Geometry: final body of the model. Coordinates: model frame, mm. A direction names the side the tool comes from. Round coordinates to 2 decimals unless told otherwise and drop trailing zeros. Loops run counter-clockwise (first coordinate to the right, second up) from the corner with the lowest first, then second, coordinate; pieces in that order, holes last. Notation, with made-up numbers: M 44.25,66.25 L 75.25,66.25 A18 cw 75.25,93.25 Z; hole C 16.5,-40 d6. An arc over 180 degrees is marked long. Answer as a JSON object with one key per item and string values.
```python
from build123d import *

# Parameters (mm, degrees)
BOSS_EXTRUDE1_DEPTH      = 30
BOSS_EXTRUDE2_DEPTH      = 14
BOSS_EXTRUDE2_DEPTH_BACK = 30
SKETCH2_W                = 14
SKETCH2_H                = 40
SKETCH3_W                = 14
SKETCH3_H                = 20
CUT_EXTRUDE1_DEPTH       = 14
CUT_EXTRUDE2_DEPTH       = 20
CUT_EXTRUDE2_DEPTH_BACK  = 20
SKETCH5_R                = 5
SKETCH6_W                = 10
SKETCH6_H                = 10
BOSS_EXTRUDE3_DEPTH      = 10
CUT_EXTRUDE3_DEPTH       = 15
CUT_EXTRUDE3_DEPTH_BACK  = 5
SKETCH7_R                = 2.5
SKETCH8_W                = 10
SKETCH8_H                = 30
BOSS_EXTRUDE4_DEPTH      = 10
SKETCH9_W                = 5
SKETCH9_H                = 30
CUT_EXTRUDE4_DEPTH       = 10
SKETCH10_R               = 10
CUT_EXTRUDE5_DEPTH       = 5
SKETCH11_R               = 12
CUT_EXTRUDE6_DEPTH       = 5
FILLET1_R                = 7
FILLET3_R                = 5
FILLET2_R                = 2.5


# Some blends are built 0.0001 mm under size
with BuildPart() as part:
    # Sketch1 → Boss-Extrude1 (new body)
    with BuildSketch(Plane(origin=(0, 0, 0), x_dir=(1, 0, 0), z_dir=(0, 1, 0))):
        with BuildLine():
            Line((0, 100), (0, 90))
            ThreePointArc((0, 90), (-90, 0), (0, -90))
            Line((0, -90), (0, -100))
            ThreePointArc((0, -100), (-100, 0), (0, 100))
        make_face()
    extrude(amount=BOSS_EXTRUDE1_DEPTH)

    # Sketch2 → Boss-Extrude2 (add, two sides: drawn at the far end of the back side and taken through both)
    with BuildSketch(Plane.XZ.offset(-BOSS_EXTRUDE2_DEPTH_BACK)):
        with Locations((-97, 0)):
            Rectangle(SKETCH2_W, SKETCH2_H)
    extrude(amount=BOSS_EXTRUDE2_DEPTH + BOSS_EXTRUDE2_DEPTH_BACK)

    # Sketch3 → Cut-Extrude1 (cut)
    with BuildSketch(Plane.XZ.offset(14)):
        with Locations((-97, 0)):
            Rectangle(SKETCH3_W, SKETCH3_H)
    extrude(amount=-CUT_EXTRUDE1_DEPTH, mode=Mode.SUBTRACT)

    # Sketch5 → Cut-Extrude2 (cut, two sides: drawn at the far end of the back side and taken through both)
    with BuildSketch(Plane.XY.offset(-CUT_EXTRUDE2_DEPTH_BACK)):
        with Locations((-97, -7)):
            Circle(SKETCH5_R)
    extrude(amount=CUT_EXTRUDE2_DEPTH + CUT_EXTRUDE2_DEPTH_BACK, mode=Mode.SUBTRACT)

    # Sketch6 → Boss-Extrude3 (add)
    with BuildSketch(Plane(origin=(0, 0, 0), x_dir=(0, 0, -1), z_dir=(1, 0, 0))):
        with Locations((95, 25)):
            Rectangle(SKETCH6_W, SKETCH6_H)
        with Locations((95, 5)):
            Rectangle(SKETCH6_W, SKETCH6_H)
    extrude(amount=BOSS_EXTRUDE3_DEPTH)

    # Sketch7 → Cut-Extrude3 (cut, two sides: drawn at the far end of the back side and taken through both)
    with BuildSketch(Plane(origin=(0, 10, 0), x_dir=(1, 0, 0), z_dir=(0, 1, 0)).offset(-CUT_EXTRUDE3_DEPTH_BACK)):
        with Locations(Location((5, 95, 0), (0, 0, 90))):
            Circle(SKETCH7_R)
    extrude(amount=CUT_EXTRUDE3_DEPTH + CUT_EXTRUDE3_DEPTH_BACK, mode=Mode.SUBTRACT)

    # Sketch8 → Boss-Extrude4 (add)
    with BuildSketch(Plane(origin=(0, 0, 0), x_dir=(0, 0, -1), z_dir=(1, 0, 0))):
        with Locations((-95, 15)):
            Rectangle(SKETCH8_W, SKETCH8_H)
    extrude(amount=BOSS_EXTRUDE4_DEPTH)

    # Sketch9 → Cut-Extrude4 (cut)
    with BuildSketch(Plane(origin=(10, 0, 0), x_dir=(0, 0, -1), z_dir=(1, 0, 0))):
        with Locations((-95, 15)):
            Rectangle(SKETCH9_W, SKETCH9_H)
    extrude(amount=-CUT_EXTRUDE4_DEPTH, mode=Mode.SUBTRACT)

    # Sketch10 → Cut-Extrude5 (cut)
    with BuildSketch(Plane.ZY.offset(104)):
        with Locations((0, 15)):
            Circle(SKETCH10_R)
    extrude(amount=-CUT_EXTRUDE5_DEPTH, mode=Mode.SUBTRACT)

    # Sketch11 → Cut-Extrude6 (cut)
    with BuildSketch(Plane.ZY.offset(99)):
        with Locations((0, 15)):
            Circle(SKETCH11_R)
    extrude(amount=-CUT_EXTRUDE6_DEPTH, mode=Mode.SUBTRACT)

    # Fillet1
    fillet1_edges = [part.edges().sort_by_distance(p)[0] for p in [
        (-104, -14, -15),
        (-90, -14, -15),
        (-104, -14, 15),
        (-90, -14, 15),
    ]]
    fillet(fillet1_edges, radius=FILLET1_R - 0.0001)  # a hair under: the kernel refuses the full size

    # Fillet3
    fillet3_edges = [part.edges().sort_by_distance(p)[0] for p in [
        (10, 5, -90),
        (10, 5, -100),
        (10, 25, -100),
        (10, 25, -90),
    ]]
    fillet(fillet3_edges, radius=FILLET3_R - 0.0001)  # a hair under: the kernel refuses the full size

    # Fillet2
    # the kernel refuses this fillet: 2.5 mm, written as the material it takes off along each edge
    with BuildSketch(Plane(origin=(0, 0, 90), x_dir=(0, 0, 1), z_dir=(1, 0, 0)), Plane(origin=(0, 30, 90), x_dir=(0, -1, 0), z_dir=(1, 0, 0))) as fillet2_piece_1:
        with BuildLine():
            CenterArc((FILLET2_R, -FILLET2_R), FILLET2_R, 90, 90)
            Line((0, -FILLET2_R), (0, 0))
            Line((0, 0), (FILLET2_R, 0))
        make_face()
    extrude(amount=16.25, mode=Mode.SUBTRACT)
    with BuildSketch(Plane(origin=(0, 0, -90), x_dir=(0, 0, -1), z_dir=(1, 0, 0)), Plane(origin=(0, 30, -90), x_dir=(0, -1, 0), z_dir=(1, 0, 0)), Plane(origin=(0, 30, -100), x_dir=(0, 0, 1), z_dir=(1, 0, 0))) as fillet2_piece_2:
        with BuildLine():
            CenterArc((FILLET2_R, FILLET2_R), FILLET2_R, 180, 90)
            Line((0, FILLET2_R), (0, 0))
            Line((0, 0), (FILLET2_R, 0))
        make_face()
    extrude(amount=5.0001, mode=Mode.SUBTRACT)
    with BuildSketch(Plane(origin=(0, 0, 0), x_dir=(0, 0, 1), z_dir=(1, 0, 0))) as fillet2_piece_3_section:
        with BuildLine():
            CenterArc((90 + FILLET2_R, -FILLET2_R), FILLET2_R, 90, 90)
            Line((90, -FILLET2_R), (90, 0))
            Line((90, 0), (90 + FILLET2_R, 0))
        make_face()
    fillet2_piece_3 = revolve(axis=Axis((0, 0, 0), (0, -1, 0)), revolution_arc=180, mode=Mode.PRIVATE)
    fillet2_piece_3 = split(fillet2_piece_3, bisect_by=Plane(origin=(-90, 0.417646948, 90.51789801), z_dir=(1, 0, 0)), keep=Keep.TOP, mode=Mode.PRIVATE)
    add(fillet2_piece_3, mode=Mode.SUBTRACT)
    with BuildSketch(Plane(origin=(0, 0, 0), x_dir=(0, 0, 1), z_dir=(1, 0, 0))) as fillet2_piece_4_section:
        with BuildLine():
            CenterArc((90 + FILLET2_R, -FILLET2_R), FILLET2_R, 90, 90)
            Line((90, -FILLET2_R), (90, 0))
            Line((90, 0), (90 + FILLET2_R, 0))
        make_face()
    fillet2_piece_4 = revolve(axis=Axis((0, 0, 0), (0, -1, 0)), revolution_arc=180, mode=Mode.PRIVATE)
    fillet2_piece_4 = split(fillet2_piece_4, bisect_by=Plane(origin=(-90.062527527, 0.003732432, 20), z_dir=(0, 0, 1)), keep=Keep.TOP, mode=Mode.PRIVATE)
    add(fillet2_piece_4, mode=Mode.SUBTRACT)
    with BuildSketch(Plane(origin=(0, 0, 0), x_dir=(0, 0, 1), z_dir=(1, 0, 0))) as fillet2_piece_5_section:
        with BuildLine():
            CenterArc((90 + FILLET2_R, -FILLET2_R), FILLET2_R, 90, 90)
            Line((90, -FILLET2_R), (90, 0))
            Line((90, 0), (90 + FILLET2_R, 0))
        make_face()
    fillet2_piece_5 = revolve(axis=Axis((0, 0, 0), (0, -1, 0)), revolution_arc=180, mode=Mode.PRIVATE)
    fillet2_piece_5 = split(fillet2_piece_5, bisect_by=Plane(origin=(-90.540406948, 0.460795961, -10), z_dir=(0, 0, 1)), keep=Keep.TOP, mode=Mode.PRIVATE)
    fillet2_piece_5 = split(fillet2_piece_5, bisect_by=Plane(origin=(-90.540406948, 0.460795961, 10), z_dir=(0, 0, -1)), keep=Keep.TOP, mode=Mode.PRIVATE)
    add(fillet2_piece_5, mode=Mode.SUBTRACT)
    with BuildSketch(Plane(origin=(0, 0, 0), x_dir=(0, 0, 1), z_dir=(1, 0, 0))) as fillet2_piece_6_section:
        with BuildLine():
            CenterArc((90 + FILLET2_R, -FILLET2_R), FILLET2_R, 90, 90)
            Line((90, -FILLET2_R), (90, 0))
            Line((90, 0), (90 + FILLET2_R, 0))
        make_face()
    fillet2_piece_6 = revolve(axis=Axis((0, 0, 0), (0, -1, 0)), revolution_arc=180, mode=Mode.PRIVATE)
    fillet2_piece_6 = split(fillet2_piece_6, bisect_by=Plane(origin=(-90.062527448, 0.003732432, -20), z_dir=(0, 0, -1)), keep=Keep.TOP, mode=Mode.PRIVATE)
    add(fillet2_piece_6, mode=Mode.SUBTRACT)
    with BuildSketch(Plane(origin=(0, 30, 0), x_dir=(0, 0, -1), z_dir=(1, 0, 0))) as fillet2_piece_7:
        with BuildLine():
            CenterArc((90 + FILLET2_R, -FILLET2_R), FILLET2_R, 90, 90)
            Line((90 + FILLET2_R, 0), (90, 0))
            Line((90, 0), (90, -FILLET2_R))
        make_face()
    revolve(axis=Axis((0, 30, 0), (0, 1, 0)), revolution_arc=180, mode=Mode.SUBTRACT)
    with BuildSketch(Plane(origin=(0, 0, 0), x_dir=(-0.9903773605712586, 0, -0.1383932211775821), z_dir=(-0.1383932211775821, 0, 0.9903773605712586))) as fillet2_piece_8_section:
        with BuildLine():
            CenterArc((100 - FILLET2_R, -FILLET2_R), FILLET2_R, 0, 90)
            Line((100, -FILLET2_R), (100, 0))
            Line((100, 0), (100 - FILLET2_R, 0))
        make_face()
    fillet2_piece_8 = revolve(axis=Axis((0, 0, 0), (0, -1, 0)), revolution_arc=82.045120461, mode=Mode.PRIVATE)
    fillet2_piece_8 = split(fillet2_piece_8, bisect_by=Plane(origin=(-62.807815321, 0.692124363, -20), z_dir=(0, 0, -1)), keep=Keep.TOP, mode=Mode.PRIVATE)
    add(fillet2_piece_8, mode=Mode.SUBTRACT)
    with BuildSketch(Plane(origin=(0, 0, -100), x_dir=(0, 0, 1), z_dir=(1, 0, 0))) as fillet2_piece_9:
        with BuildLine():
            CenterArc((FILLET2_R, -FILLET2_R), FILLET2_R, 90, 90)
            Line((0, -FILLET2_R), (0, 0))
            Line((0, 0), (FILLET2_R, 0))
        make_face()
    extrude(amount=5.0001, mode=Mode.SUBTRACT)
    with BuildSketch(Plane(origin=(5.0001, 0, -95.0001), x_dir=(1, 0, 0), z_dir=(0, 0, 1))) as fillet2_piece_10:
        with BuildLine():
            CenterArc((4.9999 - FILLET2_R, FILLET2_R), FILLET2_R, 270, 90)
            Line((4.9999, FILLET2_R), (4.9999, 0))
            Line((4.9999, 0), (4.9999 - FILLET2_R, 0))
        make_face()
    revolve(axis=Axis((5.0001, 0, -95.0001), (0, 1, 0)), revolution_arc=90, mode=Mode.SUBTRACT)
    with BuildSketch(Plane(origin=(5.0001, 0, -94.9999), x_dir=(0, 0, 1), z_dir=(-1, 0, 0))) as fillet2_piece_11:
        with BuildLine():
            CenterArc((4.9999 - FILLET2_R, FILLET2_R), FILLET2_R, 270, 90)
            Line((4.9999, FILLET2_R), (4.9999, 0))
            Line((4.9999, 0), (4.9999 - FILLET2_R, 0))
        make_face()
    revolve(axis=Axis((5.0001, 0, -94.9999), (0, 1, 0)), revolution_arc=90, mode=Mode.SUBTRACT)
    with BuildSketch(Plane(origin=(0, 30, 0), x_dir=(-0.9903773605712582, 0, -0.13839322117758568), z_dir=(-0.13839322117758568, 0, 0.9903773605712582))) as fillet2_piece_12_section:
        with BuildLine():
            CenterArc((100 - FILLET2_R, FILLET2_R), FILLET2_R, 270, 90)
            Line((100 - FILLET2_R, 0), (100, 0))
            Line((100, 0), (100, FILLET2_R))
        make_face()
    fillet2_piece_12 = revolve(axis=Axis((0, 30, 0), (0, -1, 0)), revolution_arc=82.045120461, mode=Mode.PRIVATE)
    fillet2_piece_12 = split(fillet2_piece_12, bisect_by=Plane(origin=(-62.807815321, 29.307875637, -20), z_dir=(0, 0, -1)), keep=Keep.TOP, mode=Mode.PRIVATE)
    add(fillet2_piece_12, mode=Mode.SUBTRACT)
    with BuildSketch(Plane(origin=(5.0001, 30, -95.0001), x_dir=(0, 0, -1), z_dir=(-1, 0, 0))) as fillet2_piece_13:
        with BuildLine():
            CenterArc((4.9999 - FILLET2_R, FILLET2_R), FILLET2_R, 270, 90)
            Line((4.9999, FILLET2_R), (4.9999, 0))
            Line((4.9999, 0), (4.9999 - FILLET2_R, 0))
        make_face()
    revolve(axis=Axis((5.0001, 30, -95.0001), (0, -1, 0)), revolution_arc=90, mode=Mode.SUBTRACT)
    with BuildSketch(Plane(origin=(5.0001, 30, -94.9999), x_dir=(0, 0, 1), z_dir=(-1, 0, 0))) as fillet2_piece_14:
        with BuildLine():
            CenterArc((4.9999 - FILLET2_R, -FILLET2_R), FILLET2_R, 0, 90)
            Line((4.9999, -FILLET2_R), (4.9999, 0))
            Line((4.9999, 0), (4.9999 - FILLET2_R, 0))
        make_face()
    revolve(axis=Axis((5.0001, 30, -94.9999), (0, 1, 0)), revolution_arc=90, mode=Mode.SUBTRACT)
    with BuildSketch(Plane(origin=(10, 30, -94.9999), x_dir=(-1, 0, 0), z_dir=(0, 0, -1)), Plane(origin=(10, 0, -95.0001), x_dir=(-1, 0, 0), z_dir=(0, 0, 1))) as fillet2_piece_15:
        with BuildLine():
            CenterArc((FILLET2_R, -FILLET2_R), FILLET2_R, 90, 90)
            Line((0, -FILLET2_R), (0, 0))
            Line((0, 0), (FILLET2_R, 0))
        make_face()
    extrude(amount=0.0002, mode=Mode.SUBTRACT)


solid = part.part
```
1) Line query: probe 1 along Y at (x, z) = (-97.6, 0); probe 2 along Y at (x, z) = (-101, 0); probe 3 along Z at (x, y) = (1, 4). Output: solid intervals per line, ascending.
Geometry results:
{"probe 1": "0 to 3, 27 to 30", "probe 2": "0 to 5, 25 to 30", "probe 3": "-100 to -90, 90 to 92.5, 97.5 to 100"}
2) Cut plane A-A on y = -9.5. Return the cut outline in (x, z).
Geometry results:
{"outline": "M -103.54,-20 L -101.33,-20 L -101.33,-10 L -103.54,-10 Z; M -103.54,10 L -101.33,10 L -101.33,20 L -103.54,20 Z; M -92.67,-20 L -90.46,-20 L -90.46,-10 L -92.67,-10 Z; M -92.67,10 L -90.46,10 L -90.46,20 L -92.67,20 Z"}
3) Set-up query: faces 1 (the face through (2, 6, -90)), 2 (the face through (-101.535, 24.915, -1.302)), 3 (the face through (4.9, 7.5, -92.5)), 4 (the face through (3, 10, -93)). Return all of +Z, -Z, +X, -X, +Y, -Y with unobstructed straight access to the full face (end or side cutting, diameter ignored); none if empty.
Geometry results:
{"face 1": "+X, +Y, -Y", "face 2": "-X", "face 3": "none", "face 4": "-Z, +X"}
4) First-contact query: pin 1 (19 mm diameter, centred on y = 19, z = -4.5, fed in from +X); pin 2 (5 mm diameter, centred on y = 3.5, z = -64.5, fed in from -X); pin 3 (16 mm diameter, centred on y = 15, z = 0, fed in from +X); pin 4 (11 mm diameter, centred on x = 3, y = 16.5, fed in from -Z). Flat tips, straight axial feed; report the tip coordinate or a pass-through.
Geometry results:
{"pin 1": "x = -88.9", "pin 2": "x = -78.46", "pin 3": "x = -89.64", "pin 4": "z = -100"}
5) Pull-direction query (Z, two-part tool) for faces 5 (the face through (-99, 24, -5)), 6 (the face through (-100, 8, -20)), 7 (the face through (-56, 0, -76)); classes: +Z half, -Z half, draft (parallel to the pull), parting line (faces both ways), or undercut.
Geometry results:
{"face 5": "undercut", "face 6": "-Z half", "face 7": "draft"}
6) Cut plane B-B on y = 15. Return the cut outline in (x, z), and give its area (3 significant figures).
Geometry results:
{"outline": "M -104,-20 L -97.98,-20 A100 ccw 0,-100 L 0,-90 A90 cw 0,90 L 10,90 L 10,92.5 L 0,92.5 L 0,97.5 L 10,97.5 L 10,100 L 0,100 A100 ccw -97.98,20 L -104,20 L -104,10 L -99,10 L -99,12 L -94,12 L -94,-12 L -99,-12 L -99,-10 L -104,-10 Z", "area": "3,000 mm2"}
